```python
from build123d import *

# Parameters (mm, degrees)
F1_DEPTH = 6.35
F2_DEPTH = 25.4
F0_R     = 19.05
F3_DEPTH = 50.8


# Not quite as in the source:
# - a length typed as a fraction of an inch, garbled in the dataset ("3 / 203.2 mm" for 3/8 in), is restored


with BuildPart() as f1:
    # F0 (on Top) → F1 (new body)
    with BuildSketch(Plane.XY):
        with BuildLine():
            ThreePointArc((2.54, 25.2726809025), (18.8371441572, 17.0388379885), (25.4, 0))
            Line((25.4, 0), (31.75, 0))
            ThreePointArc((31.75, 0), (33.6098719395, 4.4901280605), (38.1, 6.35))
            Line((38.1, 6.35), (88.9, 6.35))
            ThreePointArc((88.9, 6.35), (93.3901280605, 4.4901280605), (95.25, 0))
            Line((95.25, 0), (114.3, 0))
            ThreePointArc((114.3, 0), (118.4805810057, 9.4185720786), (128.27, 12.6363404513))
            Line((128.27, 12.6363404513), (2.54, 25.2726809025))
        make_face()
        with BuildLine():
            Line((31.75, 0), (25.4, 0))
            ThreePointArc((25.4, 0), (18.8371441572, -17.0388379885), (2.54, -25.2726809025))
            Line((2.54, -25.2726809025), (128.27, -12.6363404513))
            ThreePointArc((128.27, -12.6363404513), (118.4805810057, -9.4185720786), (114.3, 0))
            Line((114.3, 0), (95.25, 0))
            ThreePointArc((95.25, 0), (93.3901280605, -4.4901280605), (88.9, -6.35))
            Line((88.9, -6.35), (38.1, -6.35))
            ThreePointArc((38.1, -6.35), (33.6098719395, -4.4901280605), (31.75, 0))
        make_face()
    extrude(amount=F1_DEPTH)

    # F0 (on Top) → F2 (join)
    with BuildSketch(Plane.XY):
        with BuildLine():
            ThreePointArc((139.7, 0), (136.4185720786, 8.5194189943), (128.27, 12.6363404513))
            ThreePointArc((128.27, 12.6363404513), (118.4805810057, 9.4185720786), (114.3, 0))
            ThreePointArc((114.3, 0), (118.4805810057, -9.4185720786), (128.27, -12.6363404513))
            ThreePointArc((128.27, -12.6363404513), (136.4185720786, -8.5194189943), (139.7, 0))
        make_face()
        with BuildLine():
            ThreePointArc((133.35, 0), (127, -6.35), (120.65, 0))
            ThreePointArc((120.65, 0), (127, 6.35), (133.35, 0))
        make_face(mode=Mode.SUBTRACT)
    extrude(amount=F2_DEPTH)

    # F0 (on Top) → F3 (join)
    with BuildSketch(Plane.XY):
        with BuildLine():
            ThreePointArc((2.54, -25.2726809025), (18.8371441572, -17.0388379885), (25.4, 0))
            ThreePointArc((25.4, 0), (18.8371441572, 17.0388379885), (2.54, 25.2726809025))
            ThreePointArc((2.54, 25.2726809025), (-25.4, 0), (2.54, -25.2726809025))
        make_face()
        Circle(F0_R, mode=Mode.SUBTRACT)
    extrude(amount=F3_DEPTH)


solid = f1.part
```
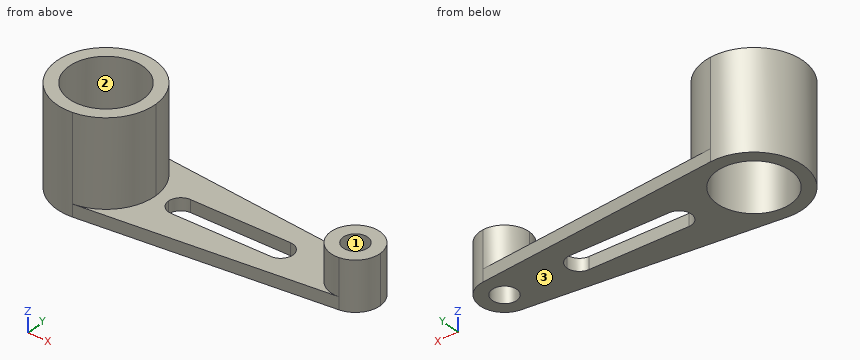
Here's how the part is built. I have some questions about the finished solid (model axes, mm). Face numbers are marked on the shaded views. Coordinates: 2 decimals unless noted, no trailing zeros. Loops run counter-clockwise (first coordinate to the right, second up) from the corner with the lowest first, then second, coordinate; pieces in that order, holes last. Notation, with made-up numbers: (-24, 23.25) - (21, 23.25) arc R14 ccw to (21, 36.25) - close; hole circle Ø2 at (89, 48). An arc over 180 degrees is marked (long way). Return JSON: item names as keys, results as strings. Group by question number.
Item 1: Will these pins go through, and if not, where does the flat tip stop? P1, Ø3, axis at x = 57, z = 2.5, coming from the -Y side; P2, Ø4, axis at y = -14.5, z = 39, coming from the -X side; P3, Ø3, axis at y = 14.5, z = 26.5, coming from the -X side.
Item 2: If we section it at D-D on y = 21.5: Write out the boundary of the cut face in (x, z), and give its area (3 significant figures).
Item 3: We'd pull the mould along X, two halves only. Please class the marked faces 1, 2 and 3: +X half, -X half, draft (parallel to the pull), parting line (faces both ways), or undercut.
Item 4: I need wall thicknesses on line 1 (Y direction, x = 0, z = 28); line 2 (X direction, y = -11, z = 11); line 3 (X direction, y = 2, z = 24). Which ranges of each line are inside material? Lowest first, please. Write a range as from..to.
Item 5: If we section it at C-C on x = 84.5: Write out the boundary of the cut face in (y, z), and give its area (3 significant figures).
Item 6: If we section it at A-A on z = 18: Write out the boundary of the cut face in (x, y), and give its area (3 significant figures).
Item 7: If we section it at B-B on x = 0: Write out the boundary of the cut face in (y, z).
Calculated:
{
 "1": {"P1": "stops at y = -19.95", "P2": "stops at x = -22.11", "P3": "stops at x = -21.82"},
 "2": {"outline": "(-13.52, 0) - (40.08, 0) - (40.08, 6.35) - (13.52, 6.35) - (13.52, 50.8) - (-13.52, 50.8) - close", "area": "1,540 mm^2"},
 "3": {"face 1": "undercut", "face 2": "undercut", "face 3": "draft"},
 "4": {"line 1": "y = -25.4..-19.05, 19.05..25.4", "line 2": "x = -22.89..-15.55, 15.55..22.89, 120.65..133.35", "line 3": "x = -25.32..-18.94, 18.94..25.32, 114.46..120.97, 133.03..139.54"},
 "5": {"outline": "(-17.04, 0) - (-6.35, 0) - (-6.35, 6.35) - (-17.04, 6.35) - close; (6.35, 0) - (17.04, 0) - (17.04, 6.35) - (6.35, 6.35) - close", "area": "136 mm^2"},
 "6": {"outline": "circle Ø50.8 at (0, 0); circle Ø25.4 at (127, 0); hole circle Ø38.1 at (0, 0); hole circle Ø12.7 at (127, 0)", "area": "1,270 mm^2"},
 "7": {"outline": "(-25.4, 0) - (-19.05, 0) - (-19.05, 50.8) - (-25.4, 50.8) - close; (19.05, 0) - (25.4, 0) - (25.4, 50.8) - (19.05, 50.8) - close"}
}
